Model file for the job. Use its own axes, mm. Face numbers are marked on the shaded views. A direction names the side the tool comes from. Give positions to 0.01 mm unless a question says otherwise; leave off trailing zeros. Order: outer loops, then holes, each group sorted by start corner. A loop starts at its lowest first (then second) coordinate and runs counter-clockwise, first axis right, second up. Notation, with made-up numbers: (49.25, 49) - (94.25, 49) arc R16 cw to (94.25, 59) - close; hole circle Ø3 at (-15.75, 23.5). An arc over 180 degrees is marked (long way). Use CSV: the item, a comma, the result in double quotes. Start each with the question number.
(1) Probe L1, parallel to Z at x = 21, y = 2; L2, parallel to Y at x = 22, z = 8.5; L3, parallel to X at y = 29.5, z = 1.75. List the from-to ranges inside material, lowest first.
(2) Drop flat-ended pins along their axis: pin 1 Ø5 at (y, z) = (27.5, 8) entering from -X; pin 2 Ø2.5 at (x, z) = (21, 11.5) entering from -Y; pin 3 Ø4 at (x, z) = (-21, 3.5) entering from +Y; pin 4 Ø5 at (y, z) = (23.5, 6) entering from +X. Give the stop position or say it passes through.
(3) Band-saw the part on D-D, the plane x = 2.5. Give the cut face in (y, z).
(4) Band-saw the part on A-A, the plane z = 3.5. Give the cut face in (x, y).
(5) Band-saw the part on B-B, the plane x = 21. Give the cut face in (y, z).
(6) Tool access for the marked faces 5, 6 and 7: list every direction of +Z, -Z, +X, -X, +Y, -Y with a clear straight run to the whole face (end or side of a thin tool).
(7) Band-saw the part on C-C, the plane z = 6.5. Give the cut face in (x, y), then the cut area to 3 significant figures.
(8) Pull direction X, two halves, no side cores. Call the marked faces 1, 2, 3 and 4: +X half, -X half, draft (parallel to the pull), parting line (faces both ways), or undercut.
from build123d import *

# Parameters (mm, degrees)
EXTRUDE_1_DEPTH     = 15
SKETCH_2_R          = 3
CUT_EXTRUDE_1_DEPTH = 45.034077713
SKETCH_3_R          = 1.5
CUT_EXTRUDE_2_DEPTH = 39.405728739
FILLET_1_R          = 1.5
CUT_EXTRUDE_3_DEPTH = 3.5


with BuildPart() as part:
    # 草图1 → 凸台-拉伸1 (new body)
    with BuildSketch(Plane.XY):
        Polygon((25, 0), (-25, 0), (-25, 8), (-15, 8), (-15, 33), (15, 33), (15, 8), (25, 8), align=None)
    extrude(amount=EXTRUDE_1_DEPTH)

    # 草图2 → 切除-拉伸1 (cut, through all)
    with BuildSketch(Plane.XY.offset(15)):
        with Locations((0, 27)):
            Circle(SKETCH_2_R)
    extrude(amount=-CUT_EXTRUDE_1_DEPTH, mode=Mode.SUBTRACT)

    # 草图3 → 切除-拉伸2 (cut, through all)
    with BuildSketch(Plane(origin=(0, 8, 0), x_dir=(1, 0, 0), z_dir=(0, 1, 0))):
        with Locations(Location((21, -3.5, 0), (0, 0, 180))):
            Circle(SKETCH_3_R)
        with Locations((21, -11.5)):
            Circle(SKETCH_3_R)
        with Locations(Location((-21, -11.5, 0), (0, 0, 180))):
            Circle(SKETCH_3_R)
        with Locations((-21, -3.5)):
            Circle(SKETCH_3_R)
    extrude(amount=-CUT_EXTRUDE_2_DEPTH, mode=Mode.SUBTRACT)

    # 圆角1
    fillet_1_edges = [part.edges().sort_by_distance(p)[0] for p in [
        (-15, 8, 7.5),
        (15, 8, 7.5),
    ]]
    fillet(fillet_1_edges, radius=FILLET_1_R)

    # 草图4 → 切除-拉伸3 (cut)
    with BuildSketch(Plane.XY.offset(15)):
        with BuildLine():
            Line((-15, 33), (-5.699842762, 22.125393094))
            ThreePointArc((-5.699842762, 22.125393094), (-7.45476136, 27.822516302), (-4.5, 33))
            Line((-4.5, 33), (-15, 33))
        make_face()
        with BuildLine():
            ThreePointArc((-5.699842762, 22.125393094), (-3.137710009, 20.1878949), (0, 19.5))
            Line((0, 19.5), (0, 24))
            ThreePointArc((0, 24), (-3, 27), (0, 30))
            Line((0, 30), (0, 33))
            Line((0, 33), (-4.5, 33))
            ThreePointArc((-4.5, 33), (-7.45476136, 27.822516302), (-5.699842762, 22.125393094))
        make_face()
        with BuildLine():
            Line((0, 24), (0, 19.5))
            ThreePointArc((0, 19.5), (3.137710009, 20.1878949), (5.699842762, 22.125393094))
            ThreePointArc((5.699842762, 22.125393094), (7.035581736, 24.401810315), (7.5, 27))
            ThreePointArc((7.5, 27), (6.708203932, 30.354101966), (4.5, 33))
            Line((4.5, 33), (0, 33))
            Line((0, 33), (0, 30))
            ThreePointArc((0, 30), (2.121320344, 29.121320344), (3, 27))
            ThreePointArc((3, 27), (2.121320344, 24.878679656), (0, 24))
        make_face()
        with BuildLine():
            ThreePointArc((7.5, 27), (7.035581736, 24.401810315), (5.699842762, 22.125393094))
            Line((5.699842762, 22.125393094), (15, 33))
            Line((15, 33), (4.5, 33))
            ThreePointArc((4.5, 33), (6.708203932, 30.354101966), (7.5, 27))
        make_face()
    extrude(amount=-CUT_EXTRUDE_3_DEPTH, mode=Mode.SUBTRACT)


solid = part.part
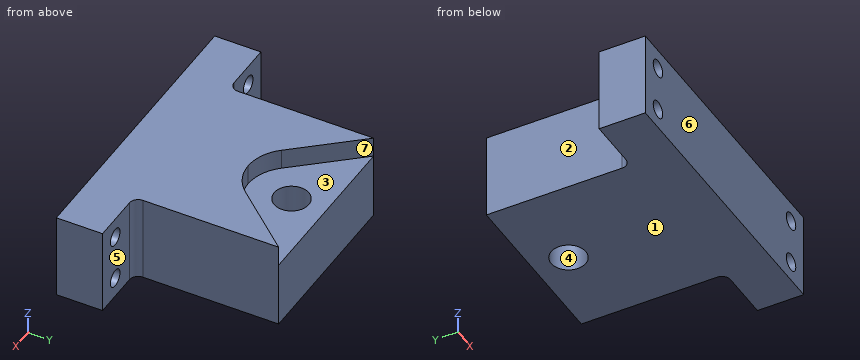
Answer block:
1,L1,"z = 0 to 2, 5 to 10, 13 to 15"
1,L2,"y = 0 to 8"
1,L3,"x = -15 to -1.66, 1.66 to 15"
2,pin 1,"stops at x = -15"
2,pin 2,"passes through"
2,pin 3,"stops at y = 8"
2,pin 4,"stops at x = 15"
3,outline,"(0, 0) - (25.34, 0) - (25.34, 11.5) - (19.93, 11.5) - (19.93, 15) - (0, 15) - close; (28.66, 0) - (33, 0) - (33, 11.5) - (28.66, 11.5) - close"
4,outline,"(-25, 0) - (-22.5, 0) - (-22.5, 8) - (-25, 8) - close; (-19.5, 0) - (19.5, 0) - (19.5, 8) - (16.5, 8) arc R1.5 cw to (15, 9.5) - (15, 33) - (-15, 33) - (-15, 9.5) arc R1.5 cw to (-16.5, 8) - (-19.5, 8) - close; (22.5, 0) - (25, 0) - (25, 8) - (22.5, 8) - close; hole circle Ø6 at (0, 27)"
5,outline,"(0, 0) - (8, 0) - (8, 2) - (0, 2) - close; (0, 5) - (8, 5) - (8, 10) - (0, 10) - close; (0, 13) - (8, 13) - (8, 15) - (0, 15) - close"
6,face 5,"+Z, -Z, +X, +Y"
6,face 6,"+Z, -Z, +X, -X, -Y"
6,face 7,"+Z, +Y"
7,outline,"(-25, 0) - (25, 0) - (25, 8) - (16.5, 8) arc R1.5 cw to (15, 9.5) - (15, 33) - (-15, 33) - (-15, 9.5) arc R1.5 cw to (-16.5, 8) - (-25, 8) - close; hole circle Ø6 at (0, 27)"
7,area,"1,120 mm2"
8,face 1,"draft"
8,face 2,"-X half"
8,face 3,"undercut"
8,face 4,"undercut"
